from build123d import *

# Parameters (mm, degrees)
SKETCH1_W           = 540
SKETCH1_H           = 170
BOSS_EXTRUDE1_DEPTH = 5
CHAMFER1_SIZE       = 1
SKETCH2_R           = 2
CUT_EXTRUDE1_DEPTH  = 5
SKETCH3_R           = 15
SKETCH3_W           = 30
SKETCH3_H           = 22
SKETCH3_W_2         = 110
SKETCH3_H_2         = 80
CUT_EXTRUDE2_DEPTH  = 10


with BuildPart() as part:
    # Sketch1 → Boss-Extrude1 (new body)
    with BuildSketch(Plane.XY):
        with Locations((270, 85)):
            Rectangle(SKETCH1_W, SKETCH1_H)
    extrude(amount=BOSS_EXTRUDE1_DEPTH)

    # Chamfer1
    chamfer1_edges = [part.edges().sort_by_distance(p)[0] for p in [
        (540, 85, 5),
        (270, 170, 5),
        (0, 85, 5),
        (270, 170, 0),
        (540, 85, 0),
        (270, 0, 0),
        (0, 85, 0),
        (0, 170, 2.5),
        (540, 170, 2.5),
        (540, 0, 2.5),
        (0, 0, 2.5),
        (270, 0, 5),
    ]]
    chamfer(chamfer1_edges, length=CHAMFER1_SIZE)

    # Sketch2 → Cut-Extrude1 (cut)
    with BuildSketch(Plane.XY.offset(5)):
        with Locations((525, 155)):
            Circle(SKETCH2_R)
        with Locations((525, 15)):
            Circle(SKETCH2_R)
        with Locations((15, 155)):
            Circle(SKETCH2_R)
        with Locations((15, 15)):
            Circle(SKETCH2_R)
    extrude(amount=-CUT_EXTRUDE1_DEPTH, mode=Mode.SUBTRACT)

    # Sketch3 → Cut-Extrude2 (cut)
    with BuildSketch(Plane(origin=(0, 0, 0), x_dir=(-1, 0, 0), z_dir=(0, 0, -1))):
        with Locations((-405, 109)):
            Circle(SKETCH3_R)
        with Locations((-455, 109)):
            Rectangle(SKETCH3_W, SKETCH3_H)
        with Locations((-125, 85)):
            Rectangle(SKETCH3_W_2, SKETCH3_H_2)
    extrude(amount=-CUT_EXTRUDE2_DEPTH, mode=Mode.SUBTRACT)


solid = part.part
Input: part model. Units: mm. Frame: model coordinates. Give positions to 0.01 mm unless a question says otherwise; leave off trailing zeros. Loops run counter-clockwise (first coordinate to the right, second up) from the corner with the lowest first, then second, coordinate; pieces in that order, holes last. Notation, with made-up numbers: M 25,46 L 80,46 A33 ccw 80,77 Z; hole C 63.5,23 d1. An arc over 180 degrees is marked long. Use CSV: the item, a comma, the result in double quotes.
(1) Section C-C, the plane z = 1.9. Return loops of the section in (x, y), plus the area to 3 significant figures.
Outcome:
outline,"M 0,1 L 1,0 L 539,0 L 540,1 L 540,169 L 539,170 L 1,170 L 0,169 Z; hole C 15,15 d4; hole C 15,155 d4; hole M 70,45 L 180,45 L 180,125 L 70,125 Z; hole C 405,109 d30; hole M 440,98 L 470,98 L 470,120 L 440,120 Z; hole C 525,15 d4; hole C 525,155 d4"
area,"81,600 mm²"
(2) Material intervals for L1, parallel to Y at x = 525, z = 3.65; L2, parallel to Y at x = 153.5, z = 2; L3, parallel to X at y = 74, z = 1.45, sorted ascending. Write a range as [from, to].
Outcome:
L1,"y = [0, 13], [17, 153], [157, 170]"
L2,"y = [0, 45], [125, 170]"
L3,"x = [0, 70], [180, 540]"
(3) Pin query (flat end, axial travel): P1, Ø5, axis at x = 525, y = 15, coming from the +Z side; P2, Ø3, axis at x = 15, y = 155, coming from the -Z side. Return the tip coordinate at first contact, or that it passes through.
Outcome:
P1,"stops at z = 5"
P2,"passes through"
(4) Section D-D, the plane x = 405. Return loops of the section in (y, z), plus the area to 3 significant figures.
Outcome:
outline,"M 0,1 L 1,0 L 94,0 L 94,5 L 1,5 L 0,4 Z; M 124,0 L 169,0 L 170,1 L 170,4 L 169,5 L 124,5 Z"
area,"698 mm²"
(5) Section A-A, the plane y = 109. Return loops of the section in (x, z).
Outcome:
outline,"M 0,1 L 1,0 L 70,0 L 70,5 L 1,5 L 0,4 Z; M 180,0 L 390,0 L 390,5 L 180,5 Z; M 420,0 L 440,0 L 440,5 L 420,5 Z; M 470,0 L 539,0 L 540,1 L 540,4 L 539,5 L 470,5 Z"
(6) Section B-B, the plane x = 77.5. Return loops of the section in (y, z).
Outcome:
outline,"M 0,1 L 1,0 L 45,0 L 45,5 L 1,5 L 0,4 Z; M 125,0 L 169,0 L 170,1 L 170,4 L 169,5 L 125,5 Z"
(7) Pull-direction query (Y, two-part tool) for faces 1 (the face through (391.144, 103.255, 2.465)), 2 (the face through (266, 86, 0)); classes: pulls with the +Y half, pulls with the -Y half, needs draft (parallel to the pull), parting line crosses it, or undercut.
Outcome:
face 1,"undercut"
face 2,"needs draft"
